CAD build for the part. Positions are in the model's coordinates, mm. A direction names the side the tool comes from. Give positions to 0.01 mm unless a question says otherwise; leave off trailing zeros. Loops run counter-clockwise (first coordinate to the right, second up) from the corner with the lowest first, then second, coordinate; pieces in that order, holes last.
Item 1: Probe probe 1 along Y at (x, z) = (0, 8.25); probe 2 along X at (y, z) = (30, 7.5); probe 3 along Y at (x, z) = (3, 12). List the from-to ranges inside material, lowest first.
Item 2: Which spindle directions (+Z, -Z, +X, -X, +Y, -Y) get a long thin tool onto all of the face, cutting with end or side? Do faces 4 (the flat face through (-5, 30, 3)), 5 (the flat face through (-6, -1, 5)), 6 (the flat face through (6, -1, 5)). Say none if no direction does.
Item 3: Saw through at B-B on z = 1.25. Give the cut face in (x, y), plus the area to 3 significant figures.
Item 4: Mould opens along X. For faces 1 (the flat face through (4.675, -1, 12)), 2 (the flat face through (-2.535, 25.69, 2.712)), 3 (the flat face through (0, -1, 13.7)) say: released by +X, released by -X, zero draft, split by the parting line, or undercut.
Item 5: Saw through at A-A on y = -30. Give the cut face in (x, z) (3 decimals).
Item 6: Saw through at C-C on y = 1. Give the cut face in (x, z) (3 decimals).
Item 7: Drop flat-ended pins along their axis: P1, Ø3.5, axis at y = -21.5, z = 11, coming from the -X side; P2, Ø0.5, axis at x = 6, y = -4.5, coming from the +Z side; P3, Ø3.5, axis at y = 13.5, z = 8.5, coming from the +X side. Give the stop position or say it passes through.
Item 8: Saw through at D-D on y = 28.5. Give the cut face in (x, z) (3 decimals).
from build123d import *

# Parameters (mm, degrees)
PAD_DEPTH       = 45
SKETCH001_R     = 3.25
POCKET_DEPTH    = 13.701
POCKET001_DEPTH = 5.5


with BuildPart() as part:
    # Sketch → Pad (new body, symmetric)
    with BuildSketch(Plane.XZ):
        Polygon((-4.675, 13.7), (4.675, 13.7), (4.675, 9.5), (5.4, 9.5), (5.4, 5), (7, 5), (7, 0), (-7, 0), (-7, 5), (-5.4, 5), (-5.4, 9.5), (-4.675, 9.5), align=None)
    extrude(amount=PAD_DEPTH, both=True)

    # Sketch001 → Pocket (cut, through all)
    with BuildSketch(Plane.XY):
        with Locations((0, -30)):
            Circle(SKETCH001_R)
        with Locations((0, 30)):
            Circle(SKETCH001_R)
    extrude(amount=POCKET_DEPTH, mode=Mode.SUBTRACT)

    # Sketch002 → Pocket001 (cut)
    with BuildSketch(Plane.XY):
        Polygon((5, 27.113249), (5, 32.886751), (0, 35.773503), (-5, 32.886751), (-5, 27.113249), (0, 24.226497), align=None)
        Polygon((0, -35.773503), (5, -32.886751), (5, -27.113249), (0, -24.226497), (-5, -27.113249), (-5, -32.886751), align=None)
    extrude(amount=POCKET001_DEPTH, mode=Mode.SUBTRACT)


solid = part.part
Results below:
1. probe 1: y = -45 to -33.25, -26.75 to 26.75, 33.25 to 45
1. probe 2: x = -5.4 to -3.25, 3.25 to 5.4
1. probe 3: y = -45 to -31.25, -28.75 to 28.75, 31.25 to 45
2. face 4: -Z
2. face 5: +Z, -X, +Y, -Y
2. face 6: +Z, +X, +Y, -Y
3. outline: (-7, -45) - (7, -45) - (7, 45) - (-7, 45) - close; hole (-5, -32.89) - (0, -35.77) - (5, -32.89) - (5, -27.11) - (0, -24.23) - (-5, -27.11) - close; hole (-5, 27.11) - (0, 24.23) - (5, 27.11) - (5, 32.89) - (0, 35.77) - (-5, 32.89) - close
3. area: 1,090 mm2
4. face 1: released by +X
4. face 2: undercut
4. face 3: zero draft
5. outline: (-7, 0) - (-5, 0) - (-5, 5.5) - (-3.25, 5.5) - (-3.25, 13.7) - (-4.675, 13.7) - (-4.675, 9.5) - (-5.4, 9.5) - (-5.4, 5) - (-7, 5) - close; (3.25, 5.5) - (5, 5.5) - (5, 0) - (7, 0) - (7, 5) - (5.4, 5) - (5.4, 9.5) - (4.675, 9.5) - (4.675, 13.7) - (3.25, 13.7) - close
6. outline: (-7, 0) - (7, 0) - (7, 5) - (5.4, 5) - (5.4, 9.5) - (4.675, 9.5) - (4.675, 13.7) - (-4.675, 13.7) - (-4.675, 9.5) - (-5.4, 9.5) - (-5.4, 5) - (-7, 5) - close
7. P1: stops at x = -5.4
7. P2: stops at z = 5
7. P3: stops at x = 5.4
8. outline: (-7, 0) - (-5, 0) - (-5, 5.5) - (-2.883, 5.5) - (-2.883, 13.7) - (-4.675, 13.7) - (-4.675, 9.5) - (-5.4, 9.5) - (-5.4, 5) - (-7, 5) - close; (2.883, 5.5) - (5, 5.5) - (5, 0) - (7, 0) - (7, 5) - (5.4, 5) - (5.4, 9.5) - (4.675, 9.5) - (4.675, 13.7) - (2.883, 13.7) - close
